```python
from build123d import *

# Parameters (mm, degrees)
F0_R     = 3.175
F1_DEPTH = 3.048


with BuildPart() as f1:
    # F0 (on Front) → F1 (new body)
    with BuildSketch(Plane.XZ):
        with BuildLine():
            ThreePointArc((-9.521768482, 60.109775595), (-6.822342257, 53.2147835566), (0, 50.3366829186))
            ThreePointArc((0, 50.3366829186), (6.7351920908, 53.1264908278), (9.525, 59.8616829186))
            ThreePointArc((9.525, 59.8616829186), (9.5212685047, 60.1282744826), (9.5100769424, 60.3946571678))
            ThreePointArc((9.5100769424, 60.3946571678), (-0.1425606912, 69.3856160057), (-9.521768482, 60.109775595))
        make_face()
        with BuildLine():
            ThreePointArc((3.175, 59.8616829186), (2.2450640303, 57.6166188883), (0, 56.6866829186))
            ThreePointArc((0, 56.6866829186), (-2.2450640303, 62.1067469488), (3.175, 59.8616829186))
        make_face(mode=Mode.SUBTRACT)
        with BuildLine():
            ThreePointArc((9.525, 59.8616829186), (6.7351920908, 53.1264908278), (0, 50.3366829186))
            Line((0, 50.3366829186), (0, 15.875))
            ThreePointArc((0, 15.875), (10.6120502723, 11.8067783082), (15.7850866092, 1.6872064905))
            Line((15.7850866092, 1.6872064905), (9.5100769424, 60.3946571678))
            ThreePointArc((9.5100769424, 60.3946571678), (9.5212685047, 60.1282744826), (9.525, 59.8616829186))
        make_face()
        with BuildLine():
            Line((0, 15.875), (0, 50.3366829186))
            ThreePointArc((0, 50.3366829186), (-6.822342257, 53.2147835566), (-9.521768482, 60.109775595))
            Line((-9.521768482, 60.109775595), (-15.7845502334, 1.6922171637))
            ThreePointArc((-15.7845502334, 1.6922171637), (-10.6101761891, 11.808462484), (0, 15.875))
        make_face()
        with Locations((-5.8420007117, 45.7200035453)):
            Circle(F0_R, mode=Mode.SUBTRACT)
        with BuildLine():
            ThreePointArc((15.7850866092, 1.6872064905), (10.6120502723, 11.8067783082), (0, 15.875))
            Line((0, 15.875), (0, 3.175))
            ThreePointArc((0, 3.175), (2.2450640303, 2.2450640303), (3.175, 0))
            ThreePointArc((3.175, 0), (2.2450640303, -2.2450640303), (0, -3.175))
            Line((0, -3.175), (0, -15.875))
            ThreePointArc((0, -15.875), (9.8507507088, -12.4490294992), (15.4497368395, -3.6498296658))
            Line((15.4497368395, -3.6498296658), (15.8561487715, -0.7734152414))
            ThreePointArc((15.8561487715, -0.7734152414), (15.8702864931, -0.3868224736), (15.875, 0))
            ThreePointArc((15.875, 0), (15.8525057155, 0.8448002958), (15.7850866092, 1.6872064905))
        make_face()
        with BuildLine():
            Line((0, 3.175), (0, 15.875))
            ThreePointArc((0, 15.875), (-10.6101761891, 11.808462484), (-15.7845502334, 1.6922171637))
            ThreePointArc((-15.7845502334, 1.6922171637), (-15.8683946878, 0.4579028636), (-15.8558659237, -0.7791924092))
            Line((-15.8558659237, -0.7791924092), (-15.4509817985, -3.644555729))
            ThreePointArc((-15.4509817985, -3.644555729), (-9.852875286, -12.4473480549), (0, -15.875))
            Line((0, -15.875), (0, -3.175))
            ThreePointArc((0, -3.175), (-3.175, 0), (0, 3.175))
        make_face()
        with BuildLine():
            Line((15.9654255085, 0), (15.7850866092, 1.6872064905))
            ThreePointArc((15.7850866092, 1.6872064905), (15.8525057155, 0.8448002958), (15.875, 0))
            ThreePointArc((15.875, 0), (15.8702864931, -0.3868224736), (15.8561487715, -0.7734152414))
            Line((15.8561487715, -0.7734152414), (15.9654255085, 0))
        make_face()
        with BuildLine():
            ThreePointArc((-15.8558659237, -0.7791924092), (-15.8683946878, 0.4579028636), (-15.7845502334, 1.6922171637))
            Line((-15.7845502334, 1.6922171637), (-15.9659680649, 0))
            Line((-15.9659680649, 0), (-15.8558659237, -0.7791924092))
        make_face()
        with BuildLine():
            Line((-15.4509817985, -3.644555729), (-15.8558659237, -0.7791924092))
            ThreePointArc((-15.8558659237, -0.7791924092), (-15.7188503178, -2.2211190167), (-15.4509817985, -3.644555729))
        make_face()
        with BuildLine():
            ThreePointArc((15.4497368395, -3.6498296658), (9.8507507088, -12.4490294992), (0, -15.875))
            Line((0, -15.875), (0, -35.3880759952))
            Line((0, -35.3880759952), (0, -41.7517314814))
            ThreePointArc((0, -41.7517314814), (2.2354081434, -42.6776678518), (3.1613445139, -44.9130759952))
            Line((3.1613445139, -44.9130759952), (9.525, -44.9130759952))
            Line((9.525, -44.9130759952), (36.5125, -44.9130759952))
            ThreePointArc((36.5125, -44.9130759952), (38.9380895153, -39.2014432113), (44.7324052746, -36.9806013807))
            Line((44.7324052746, -36.9806013807), (17.816256185, -36.0223553297))
            ThreePointArc((17.816256185, -36.0223553297), (13.8210029222, -33.4966577049), (11.8389221297, -29.2056726364))
            ThreePointArc((11.8389221297, -29.2056726364), (11.8327512172, -26.8281242675), (12.4973838852, -24.545354515))
            Line((12.4973838852, -24.545354515), (15.4497368395, -3.6498296658))
        make_face()
        with BuildLine():
            Line((0.6773435479, -35.4121902093), (0, -35.3880759952))
            ThreePointArc((0, -35.3880759952), (0.3388863295, -35.3941064578), (0.6773435479, -35.4121902093))
        make_face(mode=Mode.SUBTRACT)
        with BuildLine():
            Line((0, -35.3880759952), (0, -15.875))
            ThreePointArc((0, -15.875), (-9.852875286, -12.4473480549), (-15.4509817985, -3.644555729))
            Line((-15.4509817985, -3.644555729), (-9.4313101907, -46.2457474053))
            ThreePointArc((-9.4313101907, -46.2457474053), (-7.1909429208, -38.6667999119), (0, -35.3880759952))
        make_face()
        with BuildLine():
            ThreePointArc((15.4497368395, -3.6498296658), (15.718875865, -2.2209382121), (15.8561487715, -0.7734152414))
            Line((15.8561487715, -0.7734152414), (15.4497368395, -3.6498296658))
        make_face()
        with BuildLine():
            Line((0, -41.7517314814), (0, -35.3880759952))
            ThreePointArc((0, -35.3880759952), (-7.1909429208, -38.6667999119), (-9.4313101907, -46.2457474053))
            ThreePointArc((-9.4313101907, -46.2457474053), (-6.2462760834, -52.104018916), (0, -54.4380759952))
            Line((0, -54.4380759952), (0.6773435479, -54.4139617812))
            ThreePointArc((0.6773435479, -54.4139617812), (6.9705567315, -51.4043750835), (9.525, -44.9130759952))
            Line((9.525, -44.9130759952), (3.1613445139, -44.9130759952))
            ThreePointArc((3.1613445139, -44.9130759952), (-2.2354081434, -47.1484841387), (0, -41.7517314814))
        make_face()
        with BuildLine():
            Line((11.8389221297, -29.2056726364), (12.4973838852, -24.545354515))
            ThreePointArc((12.4973838852, -24.545354515), (11.8327512172, -26.8281242675), (11.8389221297, -29.2056726364))
        make_face()
        with BuildLine():
            Line((0.6773435479, -54.4139617812), (0, -54.4380759952))
            ThreePointArc((0, -54.4380759952), (0.3388863295, -54.4320455327), (0.6773435479, -54.4139617812))
        make_face()
        with BuildLine():
            ThreePointArc((9.525, -44.9130759952), (6.9705567315, -51.4043750835), (0.6773435479, -54.4139617812))
            Line((0.6773435479, -54.4139617812), (44.7324052746, -52.8455506098))
            ThreePointArc((44.7324052746, -52.8455506098), (38.9380895153, -50.6247087792), (36.5125, -44.9130759952))
            Line((36.5125, -44.9130759952), (9.525, -44.9130759952))
        make_face()
        with BuildLine():
            ThreePointArc((36.5125, -44.9130759952), (38.9380895153, -50.6247087792), (44.7324052746, -52.8455506098))
            ThreePointArc((44.7324052746, -52.8455506098), (50.1616327839, -50.42498648), (52.3875, -44.9130759952))
            ThreePointArc((52.3875, -44.9130759952), (50.1616327839, -39.4011655105), (44.7324052746, -36.9806013807))
            ThreePointArc((44.7324052746, -36.9806013807), (38.9380895153, -39.2014432113), (36.5125, -44.9130759952))
        make_face()
        with BuildLine():
            ThreePointArc((47.625, -44.9130759952), (44.45, -48.0880759952), (41.275, -44.9130759952))
            ThreePointArc((41.275, -44.9130759952), (44.45, -41.7380759952), (47.625, -44.9130759952))
        make_face(mode=Mode.SUBTRACT)
    extrude(amount=F1_DEPTH)


solid = f1.part
```
Design review of the part built by this model. Coordinates are the model's own, in mm. A direction names the side the tool comes from. Give positions to 0.01 mm unless a question says otherwise; leave off trailing zeros. Write each loop counter-clockwise with the first axis right and the second up, starting at its lowest first coordinate (ties: lowest second). Pieces come first, ordered by that corner, then holes. Notation, with made-up numbers: (55.25, -25.75) - (60.25, -25.75) arc R7 ccw to (60.25, -12.75) - close; hole circle Ø10 at (86.5, -23.75). An arc over 180 degrees is marked (long way). Return JSON: item names as keys, results as strings. Group by question number.
(1) To check wall thickness, follow probe 1 along Z at (x, y) = (-2.5, -0.4); probe 2 along X at (y, z) = (-2.7, -43.5); probe 3 along Z at (x, y) = (39, -0.75). State the ranges of each line that lie inside material, in increasing order.
(2) We need section A-A, the plane y = -1.15. Give the number of separate pieces and of enclosed holes in the cut face, then the cut area to 3 significant figures.
(3) Mouldability with a two-part tool opening along Z and no side actions: class faces 3 (the flat face through (3, 0, -5)), 4 (the cylindrical face through (41.517, -1.503, -46.129)), 5 (the cylindrical face through (0.061, -1.503, 69.386)) as +Z half, -Z half, draft (parallel to the pull), parting line (faces both ways), or undercut.
(4) Insertion check: pin 1 (1 mm diameter, centred on y = -1.5, z = 25.5, fed in from -X). The pin has a flat end and moves straight along its axis. Give the tip position at first contact, or say it passes through.
(5) We need section B-B, the plane z = 35. Give the boundary of the cut face in (x, y).
(6) Machinability: for faces 1 (the cylindrical face through (15.716, -1.503, -2.241)), 2 (the flat face through (-12.483, -1.503, -24.647)), which of the approach directions +Z, -Z, +X, -X, +Y, -Y give a long, thin tool a straight path to every point of the face, cutting with its end or side? Answer none if there is none.
(7) We need section C-C, the plane x = 33. Give the boundary of the cut face in (y, z).
Reported:
{
 "1": {"probe 1": "z = -54.1 to -46.85, -42.98 to -1.96, 1.96 to 57.9, 61.82 to 69.05", "probe 2": "x = -9.82 to -2.83, 2.83 to 41.61, 47.29 to 52.26", "probe 3": "z = -53.05 to -36.78"},
 "2": {"separate pieces": "1", "enclosed holes": "6", "area": "3,530 mm2"},
 "3": {"face 3": "draft", "face 4": "undercut", "face 5": "+Z half"},
 "4": {"pin 1": "stops at x = -13.29"},
 "5": {"outline": "(-12.21, -3.05) - (12.22, -3.05) - (12.22, 0) - (-12.21, 0) - close"},
 "6": {"face 1": "+X, +Y, -Y", "face 2": "-Z, -X, +Y, -Y"},
 "7": {"outline": "(-3.05, -53.26) - (0, -53.26) - (0, -36.56) - (-3.05, -36.56) - close"}
}
